Source: CAD feature listing. Evaluate the final solid. Frame: model axes, mm. Face numbers are marked on the shaded views. Round coordinates to 2 decimals unless told otherwise and drop trailing zeros. Write each loop counter-clockwise with the first axis right and the second up, starting at its lowest first coordinate (ties: lowest second). Pieces come first, ordered by that corner, then holes. Notation, with made-up numbers: M 1.25,38.25 L 25.25,38.25 A13 ccw 25.25,63.25 Z; hole C -33,-21 d5. An arc over 180 degrees is marked long. Use a Markdown table: item, result.
```python
from build123d import *

# Parameters (mm, degrees)
SCHIZZO2_R               = 4.5
TAGLIO_ESTRUSIONE1_DEPTH = 100.604216778


with BuildPart() as part:
    # Schizzo1 → Rivoluzione1 (revolve)
    with BuildSketch(Plane.XY, mode=Mode.PRIVATE) as rivoluzione1_sk:
        Polygon((0, 40), (0, 45), (-1, 45), (-1, 41.75), (-4.5, 41.75), (-4.5, 70), (-11, 70), (-11, 47.5), (-22, 47.5), (-22, 42.5), (-10, 42.5), (-10, 39), (-7, 39), (-7, 40), align=None)
    revolve(rivoluzione1_sk.sketch.rotate(Axis((-54.554939241, 0, 0), (1, 0, 0)), 90), axis=Axis((-54.554939241, 0, 0), (1, 0, 0)))

    # Schizzo2 → Taglio-Estrusione1 (cut, through all)
    with BuildSketch(Plane.ZY.offset(11)):
        with Locations((0, 60)):
            Circle(SCHIZZO2_R)
        with Locations((51.961524227, -30)):
            Circle(SCHIZZO2_R)
        with Locations((-51.961524227, -30)):
            Circle(SCHIZZO2_R)
    extrude(amount=-TAGLIO_ESTRUSIONE1_DEPTH, mode=Mode.SUBTRACT)


solid = part.part
```
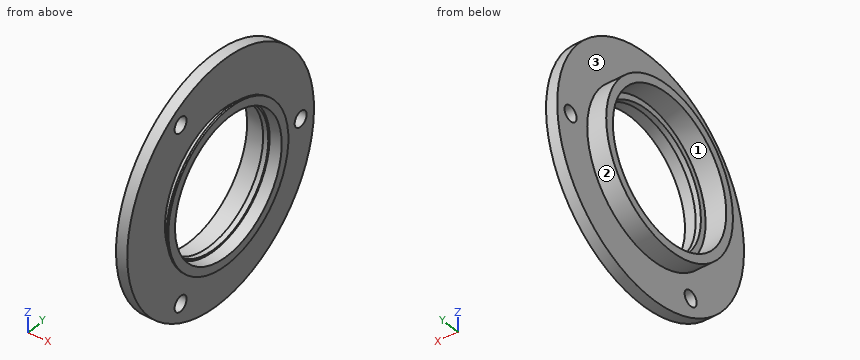
Q1. First-contact query: pin 1 Ø10 at (x, z) = (-13.5, 19) entering from -Y; pin 2 Ø1.5 at (x, z) = (-6, 35.5) entering from -Y; pin 3 Ø1.5 at (x, y) = (-9, -48.5) entering from -Z; pin 4 Ø24 at (y, z) = (-6.5, 15.5) entering from +X. Flat tips, straight axial feed; report the tip coordinate or a pass-through.
Results are:
| item | result |
|---|---|
| pin 1 | y = -68.45 |
| pin 2 | y = -60.77 |
| pin 3 | z = -51.19 |
| pin 4 | through |
Q2. Section D-D on x = -19. Return loops of the section in (y, z).
Results are:
| item | result |
|---|---|
| outline | C 0,0 d95; hole C 0,0 d85 |
Q3. Section B-B on z = 0. Give the number of separate pieces and of enclosed holes in the cut face, plus the area to 3 significant figures.
Results are:
| item | result |
|---|---|
| separate pieces | 3 |
| enclosed holes | 0 |
| area | 465 mm^2 |
Q4. Mould query, pull axis Z, two halves, no side actions, for the marked faces 1, 2 and 3. Classes: +Z half, -Z half, draft (parallel to the pull), parting line (faces both ways), or undercut.
Results are:
| item | result |
|---|---|
| face 1 | undercut |
| face 2 | parting line |
| face 3 | draft |
Q5. Section C-C on y = 28.5. Return loops of the section in (x, z).
Results are:
| item | result |
|---|---|
| outline | M -22,-38 L -11,-38 L -11,-63.94 L -4.5,-63.94 L -4.5,-30.51 L -1,-30.51 L -1,-34.82 L 0,-34.82 L 0,-28.07 L -7,-28.07 L -7,-26.62 L -10,-26.62 L -10,-31.53 L -22,-31.53 Z; M -22,31.53 L -10,31.53 L -10,26.62 L -7,26.62 L -7,28.07 L 0,28.07 L 0,34.82 L -1,34.82 L -1,30.51 L -4.5,30.51 L -4.5,63.94 L -11,63.94 L -11,38 L -22,38 Z |
Q6. Line query: L1, parallel to Y at x = -5.75, z = 0; L2, parallel to Y at x = -8.2, z = 0; L3, parallel to Z at x = -9, y = 1.5. Output: solid intervals per line, ascending.
Results are:
| item | result |
|---|---|
| L1 | -70 to -40, 40 to 55.5, 64.5 to 70 |
| L2 | -70 to -39, 39 to 55.5, 64.5 to 70 |
| L3 | -69.98 to -38.97, 38.97 to 69.98 |
Q7. Section A-A on y = 0. Return loops of the section in (x, z).
Results are:
| item | result |
|---|---|
| outline | M -22,-47.5 L -11,-47.5 L -11,-70 L -4.5,-70 L -4.5,-41.75 L -1,-41.75 L -1,-45 L 0,-45 L 0,-40 L -7,-40 L -7,-39 L -10,-39 L -10,-42.5 L -22,-42.5 Z; M -22,42.5 L -10,42.5 L -10,39 L -7,39 L -7,40 L 0,40 L 0,45 L -1,45 L -1,41.75 L -4.5,41.75 L -4.5,70 L -11,70 L -11,47.5 L -22,47.5 Z |
